```python
from build123d import *

# Parameters (mm, degrees)
SKETCH1_W               = 85.725
SKETCH1_H               = 85.725
SKETCH1_R               = 26.67
BOSS_EXTRUDE1_DEPTH     = 25.4
SKETCH2_R               = 3.572453457
CUT_EXTRUDE1_DEPTH      = 26.4
MIRROR2_COPY_1_SKETCH_R = 3.572453457
MIRROR2_COPY_1_DEPTH    = 26.4
SKETCH3_W               = 78.105
SKETCH3_H               = 78.105
CUT_EXTRUDE2_DEPTH      = 22.225
FILLET1_R               = 2.54


with BuildPart() as part:
    # Sketch1 → Boss-Extrude1 (new body)
    with BuildSketch(Plane.XY):
        Rectangle(SKETCH1_W, SKETCH1_H)
        Circle(SKETCH1_R, mode=Mode.SUBTRACT)
    extrude(amount=BOSS_EXTRUDE1_DEPTH)

    # Sketch2 → Cut-Extrude1 (cut, through all)
    with BuildSketch(Plane.XY.offset(25.4)):
        with Locations((-31.75, 31.75)):
            Circle(SKETCH2_R)
    cut_extrude1 = extrude(amount=-CUT_EXTRUDE1_DEPTH, mode=Mode.SUBTRACT)

    # Mirror1: Cut-Extrude1 across plane
    add(cut_extrude1.mirror(Plane(origin=(0, 0, 0), x_dir=(0, 0, 1), z_dir=(1, 0, 0))), mode=Mode.SUBTRACT)

    # Mirror2: Cut-Extrude1 across plane
    add(cut_extrude1.mirror(Plane.ZX), mode=Mode.SUBTRACT)

    # Mirror2 copy 1 sketch → Mirror2 copy 1 (cut, through all)
    with BuildSketch(Plane(origin=(0, 0, 25.4), x_dir=(-1, 0, 0), z_dir=(0, 0, 1))):
        with Locations((-31.75, 31.75)):
            Circle(MIRROR2_COPY_1_SKETCH_R)
    extrude(amount=-MIRROR2_COPY_1_DEPTH, mode=Mode.SUBTRACT)

    # Sketch3 → Cut-Extrude2 (cut)
    with BuildSketch(Plane(origin=(0, 0, 0), x_dir=(-1, 0, 0), z_dir=(0, 0, -1))):
        Rectangle(SKETCH3_W, SKETCH3_H)
    extrude(amount=-CUT_EXTRUDE2_DEPTH, mode=Mode.SUBTRACT)

    # Fillet1
    fillet1_edges = [part.edges().sort_by_distance(p)[0] for p in [
        (-39.0525, -39.0525, 11.1125),
        (-39.0525, 39.0525, 11.1125),
        (39.0525, 39.0525, 11.1125),
        (39.0525, -39.0525, 11.1125),
        (-42.8625, 42.8625, 12.7),
        (42.8625, 42.8625, 12.7),
        (42.8625, -42.8625, 12.7),
        (-42.8625, -42.8625, 12.7),
    ]]
    fillet(fillet1_edges, radius=FILLET1_R)


solid = part.part
```
Source: CAD feature listing. Evaluate the final solid. Frame: model axes, mm. A direction names the side the tool comes from. Coordinates: 2 decimals unless noted, no trailing zeros. Write each loop counter-clockwise with the first axis right and the second up, starting at its lowest first coordinate (ties: lowest second). Pieces come first, ordered by that corner, then holes. Notation, with made-up numbers: (18.25, 47) - (58.25, 47) arc R22 cw to (58.25, 69) - close; hole circle Ø8 at (85.25, -30). An arc over 180 degrees is marked (long way). Answer as a JSON object with one key per item and string values.
Q1. Set-up query: faces 1 (the cylindrical face through (42.099, 42.138, 12.878)), 2 (the cylindrical face through (-38.289, 38.328, 11.268)). Return all of +Z, -Z, +X, -X, +Y, -Y with unobstructed straight access to the full face (end or side cutting, diameter ignored); none if empty.
Ans:
{"face 1": "+Z, -Z, +X, +Y", "face 2": "-Z"}
Q2. Material intervals for line 1 (X direction, y = -31.75, z = 23.6); line 2 (X direction, y = 24.5, z = 4.75), sorted ascending. Write a range as [from, to].
Ans:
{"line 1": "x = [-42.86, -35.32], [-28.18, 28.18], [35.32, 42.86]", "line 2": "x = [-42.86, -39.05], [39.05, 42.86]"}
Q3. Section query D-D, the plane y = 31.75. Output: boundary loops of the cut face in (x, z) (1 decimal), plus the area to 3 significant figures.
Ans:
{"outline": "(-42.9, 0) - (-39.1, 0) - (-39.1, 22.2) - (-35.3, 22.2) - (-35.3, 25.4) - (-42.9, 25.4) - close; (-28.2, 22.2) - (28.2, 22.2) - (28.2, 25.4) - (-28.2, 25.4) - close; (35.3, 22.2) - (39.1, 22.2) - (39.1, 0) - (42.9, 0) - (42.9, 25.4) - (35.3, 25.4) - close", "area": "396 mm2"}
Q4. Section query A-A, the plane y = 0. Output: boundary loops of the cut face in (x, z) (1 decimal).
Ans:
{"outline": "(-42.9, 0) - (-39.1, 0) - (-39.1, 22.2) - (-26.7, 22.2) - (-26.7, 25.4) - (-42.9, 25.4) - close; (26.7, 22.2) - (39.1, 22.2) - (39.1, 0) - (42.9, 0) - (42.9, 25.4) - (26.7, 25.4) - close"}
Q5. Section query C-C, the plane z = 3.25. Output: boundary loops of the cut face in (x, y).
Ans:
{"outline": "(-42.86, -40.32) arc R2.54 ccw to (-40.32, -42.86) - (40.32, -42.86) arc R2.54 ccw to (42.86, -40.32) - (42.86, 40.32) arc R2.54 ccw to (40.32, 42.86) - (-40.32, 42.86) arc R2.54 ccw to (-42.86, 40.32) - close; hole (-39.05, -36.51) arc R2.54 ccw to (-36.51, -39.05) - (36.51, -39.05) arc R2.54 ccw to (39.05, -36.51) - (39.05, 36.51) arc R2.54 ccw to (36.51, 39.05) - (-36.51, 39.05) arc R2.54 ccw to (-39.05, 36.51) - close"}
Q6. First-contact query: pin 1 Ø9.5 at (x, y) = (-31.75, -31.75) entering from +Z; pin 2 Ø10 at (x, y) = (16, -30) entering from -Z (3 decimals). Flat tips, straight axial feed; report the tip coordinate or a pass-through.
Ans:
{"pin 1": "stops at z = 25.4", "pin 2": "stops at z = 22.225"}
Q7. Draft query along Y for faces 3 (the flat face through (-1, 42.862, 13)), 4 (the cylindrical face through (28.34, 32.82, 23.83)), 5 (the flat face through (-42.862, -1, 13)). Return one class per face: released by +Y, released by -Y, zero draft, split by the parting line, or undercut.
Ans:
{"face 3": "released by +Y", "face 4": "undercut", "face 5": "zero draft"}
